CAD build for the part. Positions are in the model's coordinates, mm. Face numbers are marked on the shaded views. A direction names the side the tool comes from. Coordinates: 2 decimals unless noted, no trailing zeros. Order: outer loops, then holes, each group sorted by start corner. A loop starts at its lowest first (then second) coordinate and runs counter-clockwise, first axis right, second up. Notation, with made-up numbers: (25.25, 13.5) - (59.25, 13.5) arc R31 ccw to (59.25, 50.5) - close; hole circle Ø3 at (58.5, 76). An arc over 180 degrees is marked (long way). Use one line per item in the form item = value.
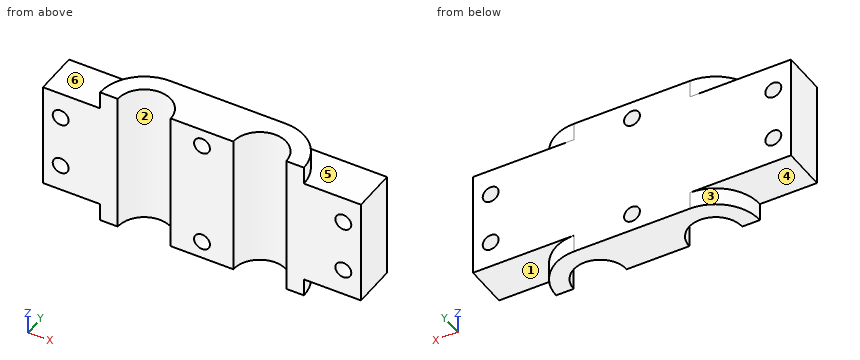
```python
from build123d import *

# Parameters (mm, degrees)
SKETCH1_W           = 90
SKETCH1_H           = 30
BOSS_EXTRUDE1_DEPTH = 6.25
BOSS_EXTRUDE3_DEPTH = 5
CUT_EXTRUDE1_DEPTH  = 41
SKETCH6_R           = 2.25
CUT_EXTRUDE2_DEPTH  = 13.5


with BuildPart() as part:
    # Sketch1 → Boss-Extrude1 (new body, symmetric)
    with BuildSketch(Plane(origin=(0, 0, 0), x_dir=(1, 0, 0), z_dir=(0, 1, 0))):
        Rectangle(SKETCH1_W, SKETCH1_H)
    extrude(amount=BOSS_EXTRUDE1_DEPTH, both=True)

    # Sketch3 → Boss-Extrude3 (add)
    with BuildSketch(Plane.XY.offset(15)):
        with BuildLine():
            Line((-28.845871038, -6.25), (-23.845871038, -6.25))
            ThreePointArc((-23.845871038, -6.25), (-16.345871038, 1.25), (-8.845871038, -6.25))
            Line((-8.845871038, -6.25), (8.845871038, -6.25))
            ThreePointArc((8.845871038, -6.25), (16.345871038, 1.25), (23.845871038, -6.25))
            Line((23.845871038, -6.25), (28.845871038, -6.25))
            ThreePointArc((28.845871038, -6.25), (25.184705803, 2.588834765), (16.345871038, 6.25))
            Line((16.345871038, 6.25), (-16.345871038, 6.25))
            ThreePointArc((-16.345871038, 6.25), (-25.184705803, 2.588834765), (-28.845871038, -6.25))
        make_face()
    boss_extrude3 = extrude(amount=BOSS_EXTRUDE3_DEPTH)

    # Mirror1: Boss-Extrude3 across plane
    add(boss_extrude3.mirror(Plane.XY))

    # Sketch5 → Cut-Extrude1 (cut)
    with BuildSketch(Plane.XY.offset(15)):
        with BuildLine():
            Line((-23.845871038, -6.25), (-8.845871038, -6.25))
            ThreePointArc((-8.845871038, -6.25), (-16.345871038, 1.25), (-23.845871038, -6.25))
        make_face()
        with BuildLine():
            Line((8.845871038, -6.25), (23.845871038, -6.25))
            ThreePointArc((23.845871038, -6.25), (16.345871038, 1.25), (8.845871038, -6.25))
        make_face()
    extrude(amount=-CUT_EXTRUDE1_DEPTH, mode=Mode.SUBTRACT)

    # Sketch6 → Cut-Extrude2 (cut, through all)
    with BuildSketch(Plane(origin=(0, 6.25, 0), x_dir=(1, 0, 0), z_dir=(0, 1, 0))):
        with Locations(Location((-40, 7.5, 0), (0, 0, 270))):  # turned: the seam where the file's is
            Circle(SKETCH6_R)
        with Locations(Location((-40, -7.5, 0), (0, 0, 270))):  # turned: the seam where the file's is
            Circle(SKETCH6_R)
        with Locations(Location((40, -7.5, 0), (0, 0, 90))):  # turned: the seam where the file's is
            Circle(SKETCH6_R)
        with Locations(Location((40, 7.5, 0), (0, 0, 90))):  # turned: the seam where the file's is
            Circle(SKETCH6_R)
        with Locations(Location((0, 15, 0), (0, 0, 270))):  # turned: the seam where the file's is
            Circle(SKETCH6_R)
        with Locations(Location((0, -15, 0), (0, 0, 90))):  # turned: the seam where the file's is
            Circle(SKETCH6_R)
    extrude(amount=-CUT_EXTRUDE2_DEPTH, mode=Mode.SUBTRACT)


solid = part.part
```
Item 1: Cut at B-B, the plane z = -7.5. Write the cut outline in (x, y).
Derived:
outline = (-45, -6.25) - (-42.25, -6.25) - (-42.25, 6.25) - (-45, 6.25) - close; (-37.75, -6.25) - (-23.85, -6.25) arc R7.5 cw to (-8.85, -6.25) - (8.85, -6.25) arc R7.5 cw to (23.85, -6.25) - (37.75, -6.25) - (37.75, 6.25) - (-37.75, 6.25) - close; (42.25, -6.25) - (45, -6.25) - (45, 6.25) - (42.25, 6.25) - close
Item 2: Cut at A-A, the plane x = 40. Write the cut outline in (y, z), plus the area to 4 significant figures.
Derived:
outline = (-6.25, -15) - (6.25, -15) - (6.25, -9.75) - (-6.25, -9.75) - close; (-6.25, -5.25) - (6.25, -5.25) - (6.25, 5.25) - (-6.25, 5.25) - close; (-6.25, 9.75) - (6.25, 9.75) - (6.25, 15) - (-6.25, 15) - close
area = 262.5 mm²
Item 3: Drop flat-ended pins along their axis: pin 1 (4 mm diameter, centred on x = -37.5, y = -1, fed in from -Z); pin 2 (6 mm diameter, centred on x = 31.5, y = 2.5, fed in from +Z). Give the stop position or say it passes through.
Derived:
pin_1 = -15
pin_2 = 15
Item 4: Drill centre lines: line 1 (X direction, y = 2, z = 7.5); line 2 (X direction, y = -4.5, z = -2.5); line 3 (Z direction, x = -1, y = 2.5). Where is each one in solid material? Low to high. Write a range as [from, to].
Derived:
line_1 = [-45, -42.25], [-37.75, 37.75], [42.25, 45]
line_2 = [-45, -23.64], [-9.05, 9.05], [23.64, 45]
line_3 = [-20, -17.02], [-12.98, 12.98], [17.02, 20]
Item 5: Cut at C-C, the plane y = 3.5. Write the cut outline in (x, z), plus the area to 3 significant figures.
Derived:
outline = (-45, -15) - (-24.17, -15) - (-24.17, -20) - (24.17, -20) - (24.17, -15) - (45, -15) - (45, 15) - (24.17, 15) - (24.17, 20) - (-24.17, 20) - (-24.17, 15) - (-45, 15) - close; hole circle Ø4.5 at (-40, -7.5); hole circle Ø4.5 at (-40, 7.5); hole circle Ø4.5 at (0, -15); hole circle Ø4.5 at (0, 15); hole circle Ø4.5 at (40, -7.5); hole circle Ø4.5 at (40, 7.5)
area = 3,090 mm²
Item 6: Cut at D-D, the plane z = -1. Write the cut outline in (x, y).
Derived:
outline = (-45, -6.25) - (-23.85, -6.25) arc R7.5 cw to (-8.85, -6.25) - (8.85, -6.25) arc R7.5 cw to (23.85, -6.25) - (45, -6.25) - (45, 6.25) - (-45, 6.25) - close
Item 7: 3-axis set-ups, long thin cutter, end or side, ignore diameter. For the marked faces 4, 5 and 6: which of +Z, -Z, +X, -X, +Y, -Y reach the whole face in a straight line?
Derived:
face_4 = -Z, -X, +Y
face_5 = +Z, +X, +Y
face_6 = +Z, -X, +Y
Item 8: Two-plate mould, pull along X, no slides. Class the marked faces 1, 2 and 3: +X half, -X half, draft (parallel to the pull), parting line (faces both ways), or undercut.
Derived:
face_1 = draft
face_2 = undercut
face_3 = -X half
